Read the model definition and answer for the solid it produces. Units are mm, in the model's axes. Face numbers are marked on the shaded views. A direction names the side the tool comes from. Coordinates: 2 decimals unless noted, no trailing zeros. Write each loop counter-clockwise with the first axis right and the second up, starting at its lowest first coordinate (ties: lowest second). Pieces come first, ordered by that corner, then holes. Notation, with made-up numbers: (55.25, -40) -> (101.25, -40) arc R21 cw to (101.25, -5) -> close; hole circle Ø10 at (38.25, 64.5). An arc over 180 degrees is marked (long way). Return JSON: item names as keys, results as strings.
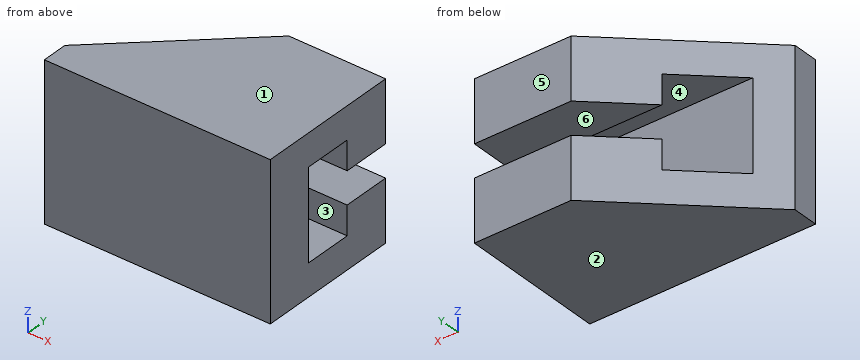
from build123d import *

# Parameters (mm, degrees)
BOSS_EXTRUDE1_DEPTH = 48
CUT_EXTRUDE1_DEPTH  = 70


with BuildPart() as part:
    # Sketch1 → Boss-Extrude1 (new body)
    with BuildSketch(Plane.XY):
        Polygon((-73.692653745, -34.694240524), (-3.692653745, -34.694240524), (-3.692653745, 10.305759476), (-33.692653745, 10.305759476), (-73.692653745, -26.694240524), align=None)
    extrude(amount=BOSS_EXTRUDE1_DEPTH)

    # Sketch2 → Cut-Extrude1 (cut)
    with BuildSketch(Plane.ZY.offset(73.692653745)):
        Polygon((19, 10.305759476), (29, 10.305759476), (29, -4.694240524), (38, -4.694240524), (38, -19.694240524), (10, -19.694240524), (10, -4.694240524), (19, -4.694240524), align=None)
    extrude(amount=-CUT_EXTRUDE1_DEPTH, mode=Mode.SUBTRACT)


solid = part.part
1. Flat-ended cylindrical pins translate along their axes: pin 1 Ø3 at (x, z) = (-35.5, 5.5) entering from +Y; pin 2 Ø1 at (y, z) = (-1.5, 33.5) entering from -X; pin 3 Ø8 at (x, z) = (-52.5, 23.5) entering from +Y; pin 4 Ø3 at (x, y) = (-47.5, 2) entering from -Z. Find the tip coordinate at first contact, or state that the pin passes through.
Taken from the geometry:
{"pin 1": "stops at y = 10.02", "pin 2": "stops at x = -47", "pin 3": "stops at y = -19.69", "pin 4": "passes through"}
2. A tool of negligible diameter and unlimited length cuts with its end or side. For the marked faces 4, 5 and 6, from which of +Z, -Z, +X, -X, +Y, -Y can it reach the whole face along a straight path? Write none if from no direction.
Taken from the geometry:
{"face 4": "+X, -X", "face 5": "+Z, -Z, +X, -X, +Y", "face 6": "+X, -X, +Y"}
3. The part is cut by section C-C (x = -10). Determine the outline of the cut face in (y, z).
Taken from the geometry:
{"outline": "(-34.69, 0) -> (10.31, 0) -> (10.31, 19) -> (-4.69, 19) -> (-4.69, 10) -> (-19.69, 10) -> (-19.69, 38) -> (-4.69, 38) -> (-4.69, 29) -> (10.31, 29) -> (10.31, 48) -> (-34.69, 48) -> close"}
4. The part is cut by section A-A (z = 13). Determine the outline of the cut face in (x, y), then the cut area to 3 significant figures.
Taken from the geometry:
{"outline": "(-73.69, -34.69) -> (-3.69, -34.69) -> (-3.69, -19.69) -> (-66.13, -19.69) -> (-73.69, -26.69) -> close; (-49.91, -4.69) -> (-3.69, -4.69) -> (-3.69, 10.31) -> (-33.69, 10.31) -> close", "area": "1,600 mm2"}
5. The part is cut by section D-D (z = 8). Determine the outline of the cut face in (x, y), then the cut area to 3 significant figures.
Taken from the geometry:
{"outline": "(-73.69, -34.69) -> (-3.69, -34.69) -> (-3.69, 10.31) -> (-33.69, 10.31) -> (-73.69, -26.69) -> close", "area": "2,410 mm2"}
6. The part is cut by section B-B (y = -13). Determine the outline of the cut face in (x, z), then the cut area to 3 significant figures.
Taken from the geometry:
{"outline": "(-58.89, 0) -> (-3.69, 0) -> (-3.69, 10) -> (-58.89, 10) -> close; (-58.89, 38) -> (-3.69, 38) -> (-3.69, 48) -> (-58.89, 48) -> close", "area": "1,100 mm2"}
7. For a pull along Z with two mould halves and no side action, classify the marked faces 1, 2 and 3 as +Z half, -Z half, draft (parallel to the pull), parting line (faces both ways), or undercut.
Taken from the geometry:
{"face 1": "+Z half", "face 2": "-Z half", "face 3": "undercut"}
8. Consider L1, parallel to Z at x = -33, y = -6.5; L2, parallel to Y at x = -61, z = 22; L3, parallel to Z at x = -17, y = 2. Determine where each line is inside the solid, lowest interval first.
Taken from the geometry:
{"L1": "z = 0 to 10, 38 to 48", "L2": "y = -34.69 to -19.69", "L3": "z = 0 to 19, 29 to 48"}
